Part print with two shaded views. Sizes in mm from the minimum x, y, z corner. A direction names the side the tool comes from. Round coordinates to 2 decimals unless told otherwise and drop trailing zeros. Write each loop counter-clockwise with the first axis right and the second up, starting at its lowest first coordinate (ties: lowest second). Pieces come first, ordered by that corner, then holes. Notation, with made-up numbers: M 68.5,-6.5 L 109.5,-6.5 A17 ccw 109.5,2.5 Z; hole C -30.75,52.5 d7. An arc over 180 degrees is marked long. One line per question, with ' | ' between items. Start each with the question number.
1) Drop flat-ended pins along their axis: pin 1 Ø5 at (x, z) = (77, 61.5) entering from -Y; pin 2 Ø10 at (x, z) = (17, 45) entering from -Y; pin 3 Ø3 at (x, y) = (90, 10.5) entering from +Z. Give the stop position or say it passes through.
2) Wall check: probe 1 along Y at (x, z) = (61, 78); probe 2 along X at (y, z) = (48, 50); probe 3 along X at (y, z) = (11.5, 18.5) (1 decimal). Give the ranges that are in metal, low to high. Write a range as [from, to].
3) Saw through at D-D (x = 93.5). List the corners of the cut face in (y, z), plus the area to 3 significant figures.
4) Saw through at B-B (y = 23). List the corners of the cut face in (x, z) (1 decimal), plus the area to 3 significant figures.
5) Mould opens along Z. For the marked faces 3, 4 and 5 say: pulls with the +Z half, pulls with the -Z half, needs draft (parallel to the pull), parting line crosses it, or undercut.
6) Saw through at A-A (z = 32.5). List the corners of the cut face in (x, y).
7) Saw through at C-C (x = 66.5). List the corners of the cut face in (y, z), plus the area to 3 significant figures.
8) Tool access for the marked faces 1 and 2: list every direction of +Z, -Z, +X, -X, +Y, -Y with a clear straight run to the whole face (end or side of a thin tool).
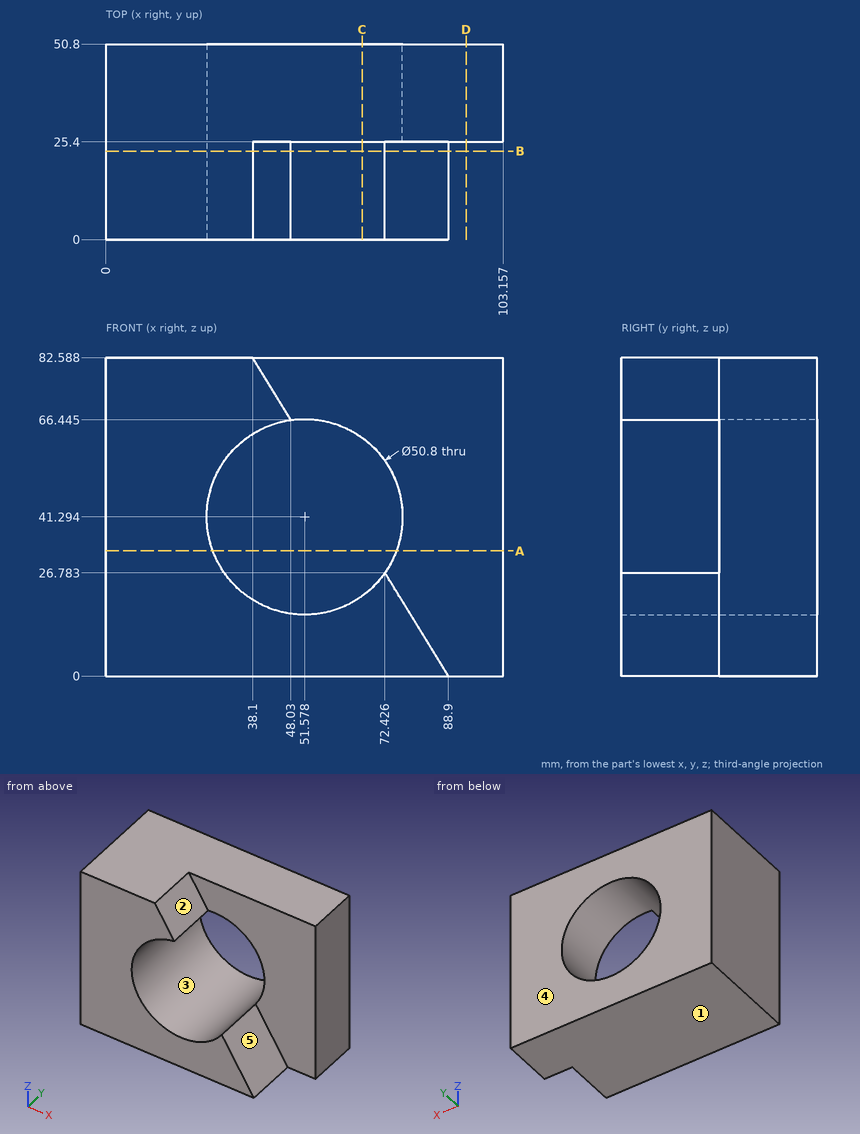
Answer key:
1) pin 1: stops at y = 25.4 | pin 2: stops at y = 0 | pin 3: stops at z = 0.65
2) probe 1: y = [25.4, 50.8] | probe 2: x = [0, 27.72], [75.44, 103.16] | probe 3: x = [0, 40.4], [62.8, 77.5]
3) outline: M 25.4,0 L 50.8,0 L 50.8,82.59 L 25.4,82.59 Z | area: 2,100 mm2
4) outline: M 0,0 L 88.9,0 L 72.4,26.8 A25.4 cw long 48,66.4 L 38.1,82.6 L 0,82.6 Z | area: 3,730 mm2
5) face 3: undercut | face 4: needs draft | face 5: pulls with the +Z half
6) outline: M 0,0 L 27.75,0 L 27.75,50.8 L 0,50.8 Z; M 75.41,25.4 L 103.16,25.4 L 103.16,50.8 L 75.41,50.8 Z
7) outline: M 0,0 L 50.8,0 L 50.8,20.74 L 0,20.74 Z; M 25.4,61.85 L 50.8,61.85 L 50.8,82.59 L 25.4,82.59 Z | area: 1,580 mm2
8) face 1: -Z, +X, -X, +Y, -Y | face 2: +Z, +X, -Y
